Could you check a few things on this drawing? It's one solid part, dimensions in mm from its lowest x, y, z. Give positions to 0.01 mm unless a question says otherwise; leave off trailing zeros. Loops run counter-clockwise (first coordinate to the right, second up) from the corner with the lowest first, then second, coordinate; pieces in that order, holes last. Notation, with made-up numbers: (57, 13.5) - (64, 13.5) arc R26 ccw to (64, 45.5) - close; hole circle Ø3 at (-32, 13). An arc over 180 degrees is marked (long way). Use a Markdown table: item, result.
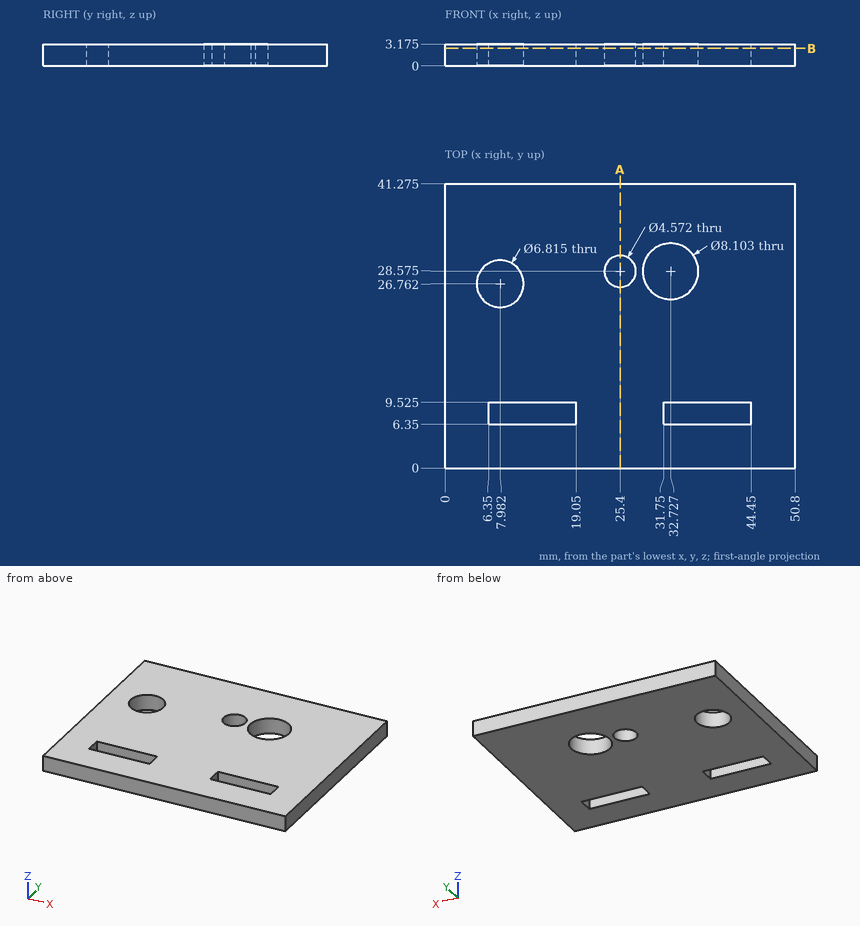
(1) Suppose I cut it at B-B on z = 2.55. Count the separate pieces of the cut face and the enclosed holes in it, plus the area to 3 significant figures.
A:
| item | result |
|---|---|
| separate pieces | 1 |
| enclosed holes | 5 |
| area | 1,910 mm2 |
(2) Will these pins go through, and if not, where does the flat tip stop? pin 1 (5 mm diameter, centred on x = 11, y = 20, fed in from -Z); pin 2 (5 mm diameter, centred on x = 32.73, y = 28.58, fed in from +Z) (3 decimals).
A:
| item | result |
|---|---|
| pin 1 | z = 0 |
| pin 2 | through |
(3) If I drill on line 1 (Y direction, x = 25.4, z = 2) (1 decimal); line 2 (X direction, y = 28, z = 1.8) (1 decimal); line 3 (X direction, y = 27, z = 1.45) (1 decimal), over which ranges is the centre line in solid material (lowest first)?
A:
| item | result |
|---|---|
| line 1 | 0 to 26.3, 30.9 to 41.3 |
| line 2 | 0 to 4.8, 11.2 to 23.2, 27.6 to 28.7, 36.7 to 50.8 |
| line 3 | 0 to 4.6, 11.4 to 23.7, 27.1 to 29, 36.5 to 50.8 |
(4) Suppose I cut it at A-A on x = 25.4. Write out the boundary of the cut face in (y, z) (1 decimal).
A:
| item | result |
|---|---|
| outline | (0, 0) - (26.3, 0) - (26.3, 3.2) - (0, 3.2) - close; (30.9, 0) - (41.3, 0) - (41.3, 3.2) - (30.9, 3.2) - close |
